Autodesk Inventor part; units mm, degrees
ref_plane "YZ Plane" through (0, 0, 0) normal (1, 0, 0) x (0, 1, 0)
ref_plane "XZ Plane" through (0, 0, 0) normal (0, 1, 0) x (-1, 0, 0)
ref_plane "XY Plane" through (0, 0, 0) normal (0, 0, 1) x (1, 0, 0)
sketch "Sketch16" plane through (0, 0, 0) normal (0, 0, 1) x (1, 0, 0)
  line L0 (-9, 5.75) -> (9, 5.75)
  line L1 (9, 5.75) -> (9, -5.75)
  line L2 (9, -5.75) -> (-9, -5.75)
  line L3 (-9, -5.75) -> (-9, 5.75)
  line L4 (-9, 5.75) -> (9, -5.75) construction
  line L5 (9, 5.75) -> (-9, -5.75) construction
  point P0 (0, 0)
  dimension "d82" = 18
  dimension "d90" = 11.5
extrude "Extrusion16" add sketch "Sketch16" along normal blind 1.75
sketch "Sketch17" plane through (0, 0, 1.75) normal (0, 0, 1) x (1, 0, 0)
  line L0 (-9, -5.75) -> (9, -5.75) construction
  line L1 (9, -5.75) -> (9, 5.75) construction
  line L2 (9, 5.75) -> (-9, 5.75) construction
  line L3 (-9, 5.75) -> (-9, -5.75) construction
  line L4 (-5.875, 5.75) -> (-1.875, 5.75)
  line L5 (-1.875, 5.75) -> (-1.875, -0.75)
  line L6 (-1.875, -0.75) -> (-5.875, -0.75)
  line L7 (-5.875, -0.75) -> (-5.875, 5.75)
  line L8 (1.875, 5.75) -> (5.875, 5.75)
  line L9 (5.875, 5.75) -> (5.875, -0.75)
  line L10 (5.875, -0.75) -> (1.875, -0.75)
  line L11 (1.875, -0.75) -> (1.875, 5.75)
  line L12 (5.875, -0.75) -> (9, -0.75) construction
  line L13 (1.875, -0.75) -> (-1.875, -0.75) construction
  line L14 (-5.875, -0.75) -> (-9, -0.75) construction
  point P0 (0, 0)
  point P1 (0, -0.75)
  dimension "d85" = 3.75
  dimension "d86" = 4
  dimension "d87" = 6.5
extrude "Extrusion17" cut sketch "Sketch17" against normal through all
properties part number "base"
The listing builds one solid part. Answer for the finished solid, in the listing's coordinates (mm). A direction names the side the tool comes from. Give positions to 0.01 mm unless a question says otherwise; leave off trailing zeros. Write each loop counter-clockwise with the first axis right and the second up, starting at its lowest first coordinate (ties: lowest second). Pieces come first, ordered by that corner, then holes. Notation, with made-up numbers: (-10, 66.25) -> (5, 66.25) arc R27 ccw to (5, 86.25) -> close; hole circle Ø11 at (-35.5, -16). An arc over 180 degrees is marked (long way). Write item = value, one per line. Start each with the question number.
1) Straight lines are drawn through the part: line 1 along X through (y, z) = (1.5, 1.65) (3 decimals); line 2 along Y through (x, z) = (2, 1.05). For each, find the intervals that lie inside material, in ascending order.
2) The part is cut by section C-C, the plane x = -3.25. Determine the outline of the cut face in (y, z).
3) Which of the six approach directions +Z, -Z, +X, -X, +Y, -Y give full straight-line access (tool end or side, diameter ignored) to faces 1 (the face through (-4, -0.75, 1)), 2 (the face through (9, 0, 1))?
4) Determine the mould class of faces 3 (the face through (-5.875, 2, 1)), 4 (the face through (-9, 0, 1)), 5 (the face through (-7, 5.75, 1)) for opening direction X: +X half, -X half, draft (parallel to the pull), parting line (faces both ways), or undercut.
5) This flat-tipped pin is pushed along its axis until it touches: pin 1 (3 mm diameter, centred on x = -4, y = 4, fed in from -Z). Where does it stop, or does it pass through?
6) The part is cut by section B-B, the plane z = 0.2. Determine the outline of the cut face in (x, y) (3 decimals).
7) The part is cut by section A-A, the plane y = 3.25. Determine the outline of the cut face in (x, z) (3 decimals).
Solutions:
q1.line_1 = -9 to -5.875, -1.875 to 1.875, 5.875 to 9
q1.line_2 = -5.75 to -0.75
q2.outline = (-5.75, 0) -> (-0.75, 0) -> (-0.75, 1.75) -> (-5.75, 1.75) -> close
q3.face_1 = +Z, -Z, +Y
q3.face_2 = +Z, -Z, +X, +Y, -Y
q4.face_3 = undercut
q4.face_4 = -X half
q4.face_5 = draft
q5.pin_1 = through
q6.outline = (-9, -5.75) -> (9, -5.75) -> (9, 5.75) -> (5.875, 5.75) -> (5.875, -0.75) -> (1.875, -0.75) -> (1.875, 5.75) -> (-1.875, 5.75) -> (-1.875, -0.75) -> (-5.875, -0.75) -> (-5.875, 5.75) -> (-9, 5.75) -> close
q7.outline = (-9, 0) -> (-5.875, 0) -> (-5.875, 1.75) -> (-9, 1.75) -> close; (-1.875, 0) -> (1.875, 0) -> (1.875, 1.75) -> (-1.875, 1.75) -> close; (5.875, 0) -> (9, 0) -> (9, 1.75) -> (5.875, 1.75) -> close
